Autodesk Inventor part; units mm, degrees
ref_plane "YZ Plane" through (0, 0, 0) normal (1, 0, 0) x (0, 1, 0)
ref_plane "XZ Plane" through (0, 0, 0) normal (0, 1, 0) x (-1, 0, 0)
ref_plane "XY Plane" through (0, 0, 0) normal (0, 0, 1) x (1, 0, 0)
sketch "Sketch1" plane through (0, 0, 0) normal (1, 0, 0) x (0, 1, 0)
  line L0 (30.0226, 0.15) -> (0.0226, 0.15)
  line L1 (0.0226, -8.075) -> (18.0226, -8.075)
  line L2 (18.0226, -8.075) -> (18.0226, -9.35)
  line L3 (18.0226, -9.35) -> (21.0226, -9.35)
  line L4 (22.0226, -3.85) -> (30.0226, -3.85)
  line L5 (30.0226, -3.85) -> (30.0226, 0.15)
  line L6 (0.0226, 0.15) -> (0.0226, -8.075)
  line L7 (50.327, 0.15) -> (-8.0634, 0.15) construction
  line L8 (22.0226, -3.85) -> (22.0226, -6.35)
  line L9 (22.0226, -6.35) -> (21.0226, -9.35)
  point P0 (0, 0)
  dimension "d0" = 4
  dimension "d2" = 3
  dimension "d4" = 8
  dimension "d5" = 30
  dimension "d7" = 8.225
  dimension "d11" = 2.5
  dimension "d12" = 1
  dimension "d14" = 0
revolve "Revolution1" add sketch "Sketch1" angle 360 about axis through (0, 50.327, 0.15) along (0, -1, 0)
fillet "Fillet1" radius 1 2 edges at (0, 21.0226, 9.65) (0, 18.0226, 9.65)
fillet "Fillet2" radius 2 1 edges at (0, 30.0226, 4.15)
fillet "Fillet3" radius 2 1 edges at (0, 0.0226, 8.375)
fillet "Fillet4" radius 2 1 edges at (0, 22.0226, 6.65)
properties part number "ConexionDireccionTop"
Can you work these out from the model? Positions are in its coordinate system, mm. A direction names the side the tool comes from. Give positions to 0.01 mm unless a question says otherwise; leave off trailing zeros. Order: outer loops, then holes, each group sorted by start corner. A loop starts at its lowest first (then second) coordinate and runs counter-clockwise, first axis right, second up. Notation, with made-up numbers: (-3, 86.5) - (9, 86.5) arc R19 ccw to (9, 91.5) - close; hole circle Ø2 at (-34, 14.5). An arc over 180 degrees is marked (long way). Use a Markdown table: item, result. Add a question column.
Q1. If we section it at A-A on y = 24.5: Write out the boundary of the cut face in (x, z).
Q2. I'm going to push flat-ended pins straight in: pin 1 (4 mm diameter, centred on y = 18, z = -5.5, fed in from -X); pin 2 (1 mm diameter, centred on x = 0, y = 21.5, fed in from +Z); pin 3 (8 mm diameter, centred on x = -0.5, z = -2.5, fed in from +Y); pin 4 (2 mm diameter, centred on x = 1.5, y = 14, fed in from +Z). Where does each tip first touch, or does it pass through?
Q3. If we section it at B-B on y = 13.25: Write out the boundary of the cut face in (x, z) (3 decimals).
Q4. Please list where these lines run through material, in increasing order: line 1 along Y through (x, z) = (-2, -0.5); line 2 along Z through (x, y) = (-0.25, 14.5); line 3 along Y through (x, z) = (-1.5, 6).
Q5. On a 3-axis mill with a long thin cutter (end or side, diameter ignored), from which of +Z, -Z, +X, -X, +Y, -Y can I reach the whole of each face in a straight line? I mean faces 1 (the cylindrical face through (8.03, 10.13, 1.93)), 2 (the cylindrical face through (8.43, 19.67, -4.23)), 3 (the flat face through (-1, 22.023, -4)). Say none if no direction works.
Answers follow:
| question | item | result |
|---|---|---|
| 1 | outline | circle Ø8 at (0, 0.15) |
| 2 | pin 1 | stops at x = -8.67 |
| 2 | pin 2 | stops at z = 9.37 |
| 2 | pin 3 | stops at y = 30.02 |
| 2 | pin 4 | stops at z = 8.36 |
| 3 | outline | circle Ø16.45 at (0, 0.15) |
| 4 | line 1 | y = 0.02 to 30.02 |
| 4 | line 2 | z = -8.07 to 8.37 |
| 4 | line 3 | y = 0.02 to 22.02 |
| 5 | face 1 | -Y |
| 5 | face 2 | +Y, -Y |
| 5 | face 3 | +Y |
